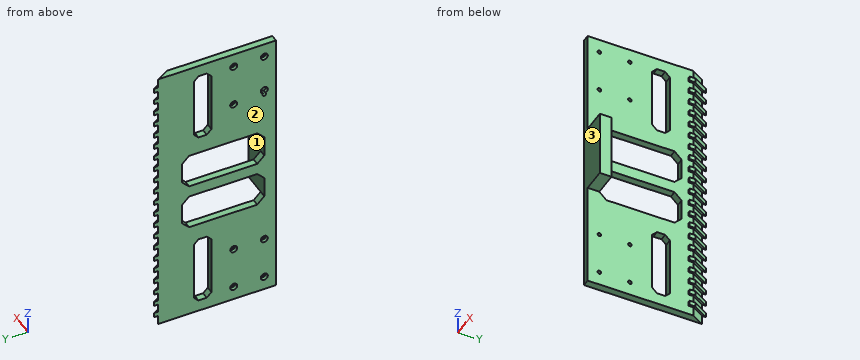
```python
from build123d import *

# Parameters (mm, degrees)
SKETCH_1_W                 = 240
SKETCH_1_H                 = 90
EXTRUDE_1_DEPTH            = 6
SKETCH_2_R                 = 1.55
CUT_EXTRUDE_1_DEPTH        = 257.390327431
SKETCH_3_W                 = 60
SKETCH_3_H                 = 15
CUT_EXTRUDE_2_DEPTH        = 257.390327431
SKETCH_4_W                 = 30
SKETCH_4_H                 = 70
CUT_EXTRUDE_3_DEPTH        = 257.390327431
SKETCH_5_R                 = 3
CUT_EXTRUDE_4_DEPTH        = 3
EXTRUDE_2_DEPTH            = 240
CHAMFER_1_SIZE             = 4
CHAMFER_2_SIZE             = 6
EXTRUDE_3_DEPTH            = 2
PATTERN_LINEAR_1_COUNT     = 11
PATTERN_LINEAR_1_PITCH     = 11
PATTERN_LINEAR_1_COL_COUNT = 11
PATTERN_LINEAR_1_COL_PITCH = 11
SKETCH_9_W                 = 57.973194975
SKETCH_9_H                 = 10
EXTRUDE_4_DEPTH            = 20


with BuildPart() as part:
    # 草图1 → 凸台-拉伸1 (new body)
    with BuildSketch(Plane(origin=(0, 0, 0), x_dir=(0, 0, -1), z_dir=(1, 0, 0))):
        with Locations((120, -45)):
            Rectangle(SKETCH_1_W, SKETCH_1_H)
    extrude(amount=EXTRUDE_1_DEPTH)

    # 草图2 → 切除-拉伸1 (cut, through all)
    with BuildSketch(Plane(origin=(6, 0, 0), x_dir=(0, 0, -1), z_dir=(1, 0, 0))):
        with Locations((12, -54)):
            Circle(SKETCH_2_R)
        with Locations((49, -80)):
            Circle(SKETCH_2_R)
        with Locations((49, -54)):
            Circle(SKETCH_2_R)
        with Locations((12, -80)):
            Circle(SKETCH_2_R)
        with Locations(Location((228, -80, 0), (0, 0, 180))):
            Circle(SKETCH_2_R)
        with Locations(Location((191, -54, 0), (0, 0, 180))):
            Circle(SKETCH_2_R)
        with Locations(Location((191, -80, 0), (0, 0, 180))):
            Circle(SKETCH_2_R)
        with Locations(Location((228, -54, 0), (0, 0, 180))):
            Circle(SKETCH_2_R)
    extrude(amount=-CUT_EXTRUDE_1_DEPTH, mode=Mode.SUBTRACT)

    # 草图3 → 切除-拉伸2 (cut, through all)
    with BuildSketch(Plane(origin=(6, 0, 0), x_dir=(0, 0, -1), z_dir=(1, 0, 0))):
        with Locations((40, -27.5)):
            Rectangle(SKETCH_3_W, SKETCH_3_H)
        with Locations((200, -27.5)):
            Rectangle(SKETCH_3_W, SKETCH_3_H)
    extrude(amount=-CUT_EXTRUDE_2_DEPTH, mode=Mode.SUBTRACT)

    # 草图4 → 切除-拉伸3 (cut, through all)
    with BuildSketch(Plane(origin=(6, 0, 0), x_dir=(0, 0, -1), z_dir=(1, 0, 0))):
        with Locations((100, -45)):
            Rectangle(SKETCH_4_W, SKETCH_4_H)
        with Locations((140, -45)):
            Rectangle(SKETCH_4_W, SKETCH_4_H)
    extrude(amount=-CUT_EXTRUDE_3_DEPTH, mode=Mode.SUBTRACT)

    # 草图5 → 切除-拉伸4 (cut)
    with BuildSketch(Plane.ZY):
        with Locations((-191, -80)):
            Circle(SKETCH_5_R)
        with Locations((-228, -80)):
            Circle(SKETCH_5_R)
        with Locations((-191, -54)):
            Circle(SKETCH_5_R)
        with Locations((-228, -54)):
            Circle(SKETCH_5_R)
        with Locations((-45, -80)):
            Circle(SKETCH_5_R)
        with Locations((-12, -80)):
            Circle(SKETCH_5_R)
        with Locations((-12, -54)):
            Circle(SKETCH_5_R)
        with Locations((-49, -54)):
            Circle(SKETCH_5_R)
    extrude(amount=-CUT_EXTRUDE_4_DEPTH, mode=Mode.SUBTRACT)

    # 草图6 → 凸台-拉伸2 (add)
    with BuildSketch(Plane.XY):
        Polygon((6, 0), (0, 0), (0, 10.392304845), align=None)
    extrude(amount=-EXTRUDE_2_DEPTH)

    # 倒角1
    chamfer_1_edges = [part.edges().sort_by_distance(p)[0] for p in [
        (3, -35, -10),
        (3, -20, -10),
        (3, -20, -70),
        (3, -35, -70),
        (3, -20, -170),
        (3, -20, -230),
        (3, -35, -230),
        (3, -35, -170),
    ]]
    chamfer(chamfer_1_edges, length=CHAMFER_1_SIZE)

    # 倒角2
    chamfer_2_edges = [part.edges().sort_by_distance(p)[0] for p in [
        (3, -10, -115),
        (3, -80, -115),
        (3, -80, -85),
        (3, -10, -85),
        (3, -10, -125),
        (3, -10, -155),
        (3, -80, -155),
        (3, -80, -125),
    ]]
    chamfer(chamfer_2_edges, length=CHAMFER_2_SIZE)

    # 草图8 → 凸台-拉伸3 (add, symmetric)
    with BuildSketch(Plane.XY.offset(-120)):
        Polygon((0, 10.392304845), (0, 13.892304845), (7.5, 0.901923789), (7.5, -4), (6, -4), (6, 0), align=None)
    extrude_3 = extrude(amount=EXTRUDE_3_DEPTH, both=True)

    # 阵列(线性)1: 凸台-拉伸3 ×11
    with Locations(*[(0, 0, i * PATTERN_LINEAR_1_PITCH) for i in range(1, PATTERN_LINEAR_1_COUNT)]):
        add(extrude_3)

    # 阵列(线性)1 col: 凸台-拉伸3 ×11
    with Locations(*[(0, 0, -i * PATTERN_LINEAR_1_COL_PITCH) for i in range(1, PATTERN_LINEAR_1_COL_COUNT)]):
        add(extrude_3)

    # 草图9 → 凸台-拉伸4 (add)
    with BuildSketch(Plane(origin=(6, 0, 0), x_dir=(0, 0, -1), z_dir=(1, 0, 0))):
        with Locations((119.986597488, -85)):
            Rectangle(SKETCH_9_W, SKETCH_9_H)
    extrude(amount=EXTRUDE_4_DEPTH)


solid = part.part
```
Can you work these out from the model? Positions are in its coordinate system, mm. Face numbers are marked on the shaded views. Give positions to 0.01 mm unless a question says otherwise; leave off trailing zeros. Loops run counter-clockwise (first coordinate to the right, second up) from the corner with the lowest first, then second, coordinate; pieces in that order, holes last. Notation, with made-up numbers: M -24,74.25 L 22,74.25 A12 cw 22,97.25 Z; hole C 67,-21 d8. An arc over 180 degrees is marked long. One line per question, with ' | ' between items. Start each with the question number.
Q1. If we section it at B-B (x = 16.25): Please give me the cut outline in (y, z), plus the area to 3 significant figures.
Q2. For pin 1 Ø2 at (x, z) = (18.5, -121) entering from +Y; pin 2 Ø4.5 at (y, z) = (-1, -143) entering from +X; pin 3 Ø10 at (x, z) = (12, -108.5) entering from +Y, each with a flat end and sliding along its axis, tell me the tip position at first contact or that it passes through.
Q3. If we mould it in two halves opening along Y, with no side actions, what happens to the marked faces 1, 2 and 3? For each: +Y half, -Y half, draft (parallel to the pull), parting line (faces both ways), or undercut.
Q4. If I drill on line 1 (Y direction, x = 5.5, z = -24); line 2 (Z direction, x = 1.5, y = -75); line 3 (Z direction, x = 2.75, y = -46), over which ranges is the centre line in solid material (lowest first)? Write a range as from..to.
Q5. If we section it at A-A (z = -26): Please give me the cut outline in (x, y), plus the area to 3 significant figures.
Computed:
1) outline: M -90,-148.97 L -80,-148.97 L -80,-91 L -90,-91 Z | area: 580 mm²
2) pin 1: stops at y = -80 | pin 2: stops at x = 7.5 | pin 3: stops at y = 1.77
3) face 1: undercut | face 2: draft | face 3: -Y half
4) line 1: y = -90..-35, -20..0.87 | line 2: z = -240..-154, -126..-114, -86..0 | line 3: z = -240..-155, -125..-115, -85..0
5) outline: M 0,-90 L 6,-90 L 6,-35 L 0,-35 Z; M 0,-20 L 6,-20 L 6,0 L 0,10.39 Z | area: 481 mm²
